Could you check a few things on this drawing? It's one solid part, dimensions in mm from its lowest x, y, z. A direction names the side the tool comes from. Coordinates: 2 decimals unless noted, no trailing zeros. Order: outer loops, then holes, each group sorted by start corner. A loop starts at its lowest first (then second) coordinate and runs counter-clockwise, first axis right, second up.
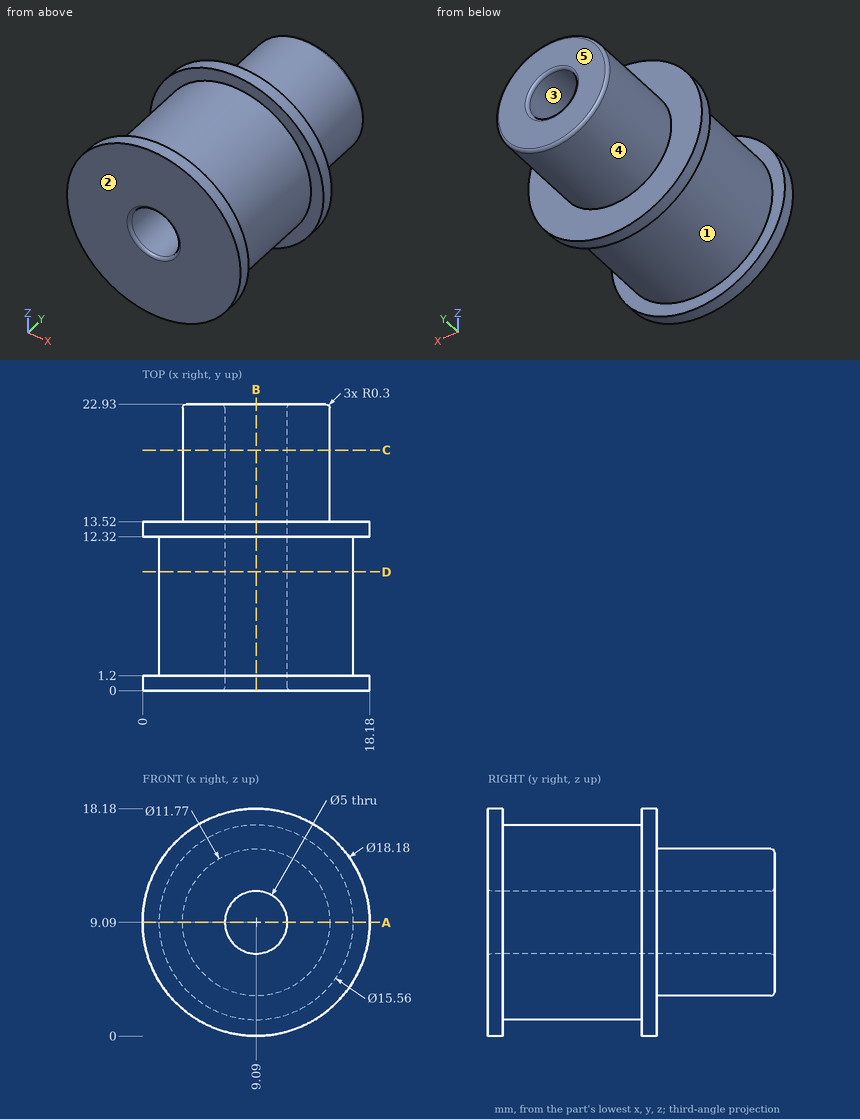
Item 1: Suppose I cut it at C-C (y = 19.25). List the corners of the cut face in (x, z) for me (3 decimals).
Item 2: For pin 1 Ø1.5 at (y, z) = (19, 6.5) entering from -X; pin 2 Ø4 at (y, z) = (9.5, 12.5) entering from +X; pin 3 Ø4 at (y, z) = (9.5, 6) entering from -X, each with a flat end and sliding along its axis, tell me the tip position at first contact or that it passes through.
Item 3: Suppose I cut it at A-A (z = 9.09). List the corners of the cut face in (x, y) for me (3 decimals), and give its area (3 significant figures).
Item 4: Suppose I cut it at B-B (x = 9.09). List the corners of the cut face in (y, z) for me (3 decimals).
Item 5: Which directions (+Z, -Z, +X, -X, +Y, -Y) give clear straight access to the entire face, cutting with the end or side of a thin tool? Please do the marked faces 4 and 5.
Item 6: Thinking about a two-plate mould opening in X: for the marked faces 1, 2 and 3, which applies, +X half, -X half, draft (parallel to the pull), parting line (faces both ways), or undercut?
Item 7: Suppose I cut it at D-D (y = 9.5). List the corners of the cut face in (x, z) for me.
Item 8: I need wall thicknesses on line 1 (Z direction, x = 9.09, y = 18) (3 decimals); line 2 (Y direction, x = 15.5, z = 3.5); line 3 (Z direction, x = 9.09, y = 9.25). Which ranges of each line are inside material? Lowest first, please.
Geometry results:
1. outline: circle Ø11.77 at (9.09, 9.09); hole circle Ø5 at (9.09, 9.09)
2. pin 1: stops at x = 3.5
2. pin 2: stops at x = 16.74
2. pin 3: stops at x = 1.39
3. outline: (0, 0) - (6.29, 0) arc R0.3 ccw to (6.59, 0.3) - (6.59, 22.63) arc R0.3 ccw to (6.29, 22.93) - (3.505, 22.93) arc R0.3 ccw to (3.205, 22.63) - (3.205, 13.52) - (0, 13.52) - (0, 12.32) - (1.31, 12.32) - (1.31, 1.2) - (0, 1.2) - close; (11.59, 0.3) arc R0.3 ccw to (11.89, 0) - (18.18, 0) - (18.18, 1.2) - (16.87, 1.2) - (16.87, 12.32) - (18.18, 12.32) - (18.18, 13.52) - (14.975, 13.52) - (14.975, 22.63) arc R0.3 ccw to (14.675, 22.93) - (11.89, 22.93) arc R0.3 ccw to (11.59, 22.63) - close
3. area: 213 mm2
4. outline: (0, 0) - (1.2, 0) - (1.2, 1.31) - (12.32, 1.31) - (12.32, 0) - (13.52, 0) - (13.52, 3.205) - (22.63, 3.205) arc R0.3 ccw to (22.93, 3.505) - (22.93, 6.29) arc R0.3 ccw to (22.63, 6.59) - (0.3, 6.59) arc R0.3 ccw to (0, 6.29) - close; (0, 11.89) arc R0.3 ccw to (0.3, 11.59) - (22.63, 11.59) arc R0.3 ccw to (22.93, 11.89) - (22.93, 14.675) arc R0.3 ccw to (22.63, 14.975) - (13.52, 14.975) - (13.52, 18.18) - (12.32, 18.18) - (12.32, 16.87) - (1.2, 16.87) - (1.2, 18.18) - (0, 18.18) - close
5. face 4: +Y
5. face 5: +Z, -Z, +X, -X, +Y
6. face 1: parting line
6. face 2: draft
6. face 3: undercut
7. outline: circle Ø15.56 at (9.09, 9.09); hole circle Ø5 at (9.09, 9.09)
8. line 1: z = 3.205 to 6.59, 11.59 to 14.975
8. line 2: y = 0 to 1.2, 12.32 to 13.52
8. line 3: z = 1.31 to 6.59, 11.59 to 16.87
